Design review of the part built by this model. Coordinates are the model's own, in mm. A direction names the side the tool comes from. Give positions to 0.01 mm unless a question says otherwise; leave off trailing zeros. Loops run counter-clockwise (first coordinate to the right, second up) from the corner with the lowest first, then second, coordinate; pieces in that order, holes last. Notation, with made-up numbers: M 3,76 L 15,76 A20 ccw 15,91 Z; hole C 81.25,45.25 d11. An arc over 180 degrees is marked long. Use CSV: the item, a comma, the result in double quotes.
from build123d import *

# Parameters (mm, degrees)
BASE_EXTRUDE_DEPTH = 101.6
HOLE1_START        = -18.5166
HOLE1_OUTLINE_R    = 7.14375
HOLE1_DEPTH        = 1.4986
LPATTERN2_COUNT    = 2
LPATTERN2_PITCH    = 47.625


# Read off the part's stored shape, not the designer's step: Hole1
with BuildPart() as part:
    # Sketch1 → Base-Extrude (new body)
    with BuildSketch(Plane.XY):
        with BuildLine():
            Line((17.6403, 16.339286512), (19.729882578, 19.063533504))
            ThreePointArc((19.729882578, 19.063533504), (19.156045845, 20.609744632), (17.6403, 21.2598))
            Line((17.6403, 21.2598), (14.70327367, 21.2598))
            ThreePointArc((14.70327367, 21.2598), (13.223883481, 20.647016519), (12.6111, 19.16762633))
            Line((12.6111, 19.16762633), (12.6111, 15.61465))
            Line((12.6111, 15.61465), (11.1125, 15.61465))
            Line((11.1125, 15.61465), (11.1125, 19.16762633))
            ThreePointArc((11.1125, 19.16762633), (12.164213258, 21.706686742), (14.70327367, 22.7584))
            Line((14.70327367, 22.7584), (17.6403, 22.7584))
            ThreePointArc((17.6403, 22.7584), (20.415434554, 21.446284653), (21.162428673, 18.4688666))
            Line((21.162428673, 18.4688666), (19.1389, 15.830735923))
            Line((19.1389, 15.830735923), (19.1389, 10.749129415))
            Line((19.1389, 10.749129415), (20.6375, 9.0662125))
            Line((20.6375, 9.0662125), (20.6375, -4.8244125))
            Line((20.6375, -4.8244125), (19.1389, -6.507329415))
            Line((19.1389, -6.507329415), (19.1389, -13.358784555))
            Line((19.1389, -13.358784555), (20.553458003, -14.773342558))
            ThreePointArc((20.553458003, -14.773342558), (18.729942105, -18.270236732), (15.019825564, -16.932883251))
            ThreePointArc((15.019825564, -16.932883251), (13.000752562, -16.523120627), (12.480559153, -18.5166))
            Line((12.480559153, -18.5166), (-12.480559153, -18.5166))
            ThreePointArc((-12.480559153, -18.5166), (-13.000752562, -16.523120627), (-15.019825564, -16.932883251))
            ThreePointArc((-15.019825564, -16.932883251), (-18.729942105, -18.270236732), (-20.553458003, -14.773342558))
            Line((-20.553458003, -14.773342558), (-19.1389, -13.358784555))
            Line((-19.1389, -13.358784555), (-19.1389, -6.507329415))
            Line((-19.1389, -6.507329415), (-20.6375, -4.8244125))
            Line((-20.6375, -4.8244125), (-20.6375, 9.0662125))
            Line((-20.6375, 9.0662125), (-19.1389, 10.749129415))
            Line((-19.1389, 10.749129415), (-19.1389, 15.830735923))
            Line((-19.1389, 15.830735923), (-21.162428673, 18.4688666))
            ThreePointArc((-21.162428673, 18.4688666), (-20.415434554, 21.446284653), (-17.6403, 22.7584))
            Line((-17.6403, 22.7584), (-14.70327367, 22.7584))
            ThreePointArc((-14.70327367, 22.7584), (-12.164213258, 21.706686742), (-11.1125, 19.16762633))
            Line((-11.1125, 19.16762633), (-11.1125, 15.61465))
            Line((-11.1125, 15.61465), (-12.6111, 15.61465))
            Line((-12.6111, 15.61465), (-12.6111, 19.16762633))
            ThreePointArc((-12.6111, 19.16762633), (-13.223883481, 20.647016519), (-14.70327367, 21.2598))
            Line((-14.70327367, 21.2598), (-17.6403, 21.2598))
            ThreePointArc((-17.6403, 21.2598), (-19.156045845, 20.609744632), (-19.729882578, 19.063533504))
            Line((-19.729882578, 19.063533504), (-17.6403, 16.339286512))
            Line((-17.6403, 16.339286512), (-17.6403, 10.17860201))
            Line((-17.6403, 10.17860201), (-19.1389, 8.495685095))
            Line((-19.1389, 8.495685095), (-19.1389, -4.253885095))
            Line((-19.1389, -4.253885095), (-17.6403, -5.93680201))
            Line((-17.6403, -5.93680201), (-17.6403, -13.979525))
            Line((-17.6403, -13.979525), (-19.1389, -15.478125))
            ThreePointArc((-19.1389, -15.478125), (-18.092238669, -16.906954381), (-16.414285827, -16.33992034))
            ThreePointArc((-16.414285827, -16.33992034), (-13.428073412, -14.819877156), (-10.898992189, -17.018))
            Line((-10.898992189, -17.018), (10.898992189, -17.018))
            ThreePointArc((10.898992189, -17.018), (13.323359075, -14.834630878), (16.30518861, -16.15877141))
            ThreePointArc((16.30518861, -16.15877141), (17.990302879, -16.935279743), (19.1389, -15.478125))
            Line((19.1389, -15.478125), (17.6403, -13.979525))
            Line((17.6403, -13.979525), (17.6403, -5.93680201))
            Line((17.6403, -5.93680201), (19.1389, -4.253885095))
            Line((19.1389, -4.253885095), (19.1389, 8.495685095))
            Line((19.1389, 8.495685095), (17.6403, 10.17860201))
            Line((17.6403, 10.17860201), (17.6403, 16.339286512))
        make_face()
    extrude(amount=BASE_EXTRUDE_DEPTH)

    # Hole1 outline → Hole1 (cut)
    with BuildSketch(Plane(origin=(0, 0, 0), x_dir=(1, 0, 0), z_dir=(0, 1, 0)).offset(HOLE1_START)):
        with Locations((0, -23.8125)):
            Circle(HOLE1_OUTLINE_R)
    hole1 = extrude(amount=HOLE1_DEPTH, mode=Mode.SUBTRACT)

    # LPattern2: Hole1 ×2
    with Locations(*[(0, 0, i * LPATTERN2_PITCH) for i in range(1, LPATTERN2_COUNT)]):
        add(hole1, mode=Mode.SUBTRACT)


solid = part.part
(1) The part is to be moulded in two halves that separate along Y. For faces 1 (the flat face through (19.139, 13, 50)), 2 (the flat face through (16, 22.758, 50)), 3 (the cylindrical face through (-0.93, -17.778, 64.355)), 4 (the flat face through (0, -18.517, 50)), say which applies: released by +Y, released by -Y, zero draft, split by the parting line, or undercut.
A:
face 1,"undercut"
face 2,"released by +Y"
face 3,"zero draft"
face 4,"released by -Y"
(2) Wall thickness on line 1 along X through (y, z) = (8, 80); line 2 along Y through (x, z) = (17.5, 73); line 3 along X through (y, z) = (-12, 47): over which ranges is each line inside the solid? List them lowest first. Write a range as [from, to].
A:
line 1,"[-20.64, -19.14], [19.14, 20.64]"
line 2,"[-18.47, -16.97], [21.26, 22.76]"
line 3,"[-19.14, -17.64], [17.64, 19.14]"
(3) We need section B-B on x = 8.5. State the section outline as (y, z) points.
A:
outline,"M -18.52,0 L -17.02,0 L -17.02,101.6 L -18.52,101.6 Z"
(4) We need section A-A on x = 0. State the section outline as (y, z) points.
A:
outline,"M -18.52,0 L -17.02,0 L -17.02,16.67 L -18.52,16.67 Z; M -18.52,30.96 L -17.02,30.96 L -17.02,64.29 L -18.52,64.29 Z; M -18.52,78.58 L -17.02,78.58 L -17.02,101.6 L -18.52,101.6 Z"
(5) Clearance check with flat-ended pins moving along their axes: P1, Ø15.5, axis at y = -1, z = 55.5, coming from the +X side; P2, Ø11.5, axis at x = 0, z = 23.81, coming from the -Y side; P3, Ø4, axis at y = -10.5, z = 37.5, coming from the -X side; P4, Ø7, axis at y = 3, z = 64, coming from the -X side. State where each tip first meets the part, or that it passes through.
A:
P1,"x = 20.64"
P2,"through"
P3,"x = -19.14"
P4,"x = -20.64"
(6) Machinability: for faces 5 (the cylindrical face through (17.963, -16.942, 50.089)), 6 (the flat face through (-20.638, 2, 50)), 7 (the flat face through (-19.139, 13, 50)), 8 (the flat face through (19.139, -10, 50)), 9 (the flat face through (-11.112, 17, 50)), which of the approach directions +Z, -Z, +X, -X, +Y, -Y give a long, thin tool a straight path to every point of the face, cutting with its end or side? Answer none if there is none.
A:
face 5,"+Z, -Z"
face 6,"+Z, -Z, -X, -Y"
face 7,"+Z, -Z, -X"
face 8,"+Z, -Z, +X"
face 9,"+Z, -Z, +Y"
